Build history of the part. All positions in model axes, mm. Face numbers are marked on the shaded views. A direction names the side the tool comes from. Round coordinates to 2 decimals unless told otherwise and drop trailing zeros. Order: outer loops, then holes, each group sorted by start corner. A loop starts at its lowest first (then second) coordinate and runs counter-clockwise, first axis right, second up. Notation, with made-up numbers: M 55.5,-30 L 100.5,-30 A27 cw 100.5,3 Z; hole C 16.5,-40 d1. An arc over 180 degrees is marked long. One line per item, written item: value. Start each with the question number.
Item 1: Band-saw the part on B-B, the plane x = -107.95. Write the cut outline in (y, z) (3 decimals), then the cut area to 3 significant figures.
Item 2: Two-plate mould, pull along X, no slides. Class the marked faces 6, 7 and 8: +X half, -X half, draft (parallel to the pull), parting line (faces both ways), or undercut.
Item 3: Tool access for the marked faces 1, 2, 3, 4 and 5: list every direction of +Z, -Z, +X, -X, +Y, -Y with a clear straight run to the whole face (end or side of a thin tool).
Item 4: Band-saw the part on D-D, the plane y = 23.5. Write the cut outline in (x, z).
Item 5: Probe L1, parallel to X at y = 203, z = 29; L2, parallel to Y at x = -107.95, z = 28 (3 decimals); L3, parallel to X at y = 208, z = 11. List the from-to ranges inside material, lowest first.
Item 6: Band-saw the part on A-A, the plane y = 203.2. Write the cut outline in (x, z) (3 decimals), then the cut area to 3 significant figures.
Item 7: Pin check, flat tips, straight feed: pin 1 (19 mm diameter, centred on x = 10.5, z = 14.5, fed in from -Y); pin 2 (6 mm diameter, centred on x = -39, z = 7.5, fed in from +Y); pin 3 (1.5 mm diameter, centred on y = 55.5, z = 26.5, fed in from -X). Stop position of each tip, or through.
Item 8: Band-saw the part on C-C, the plane z = 21. Write the cut outline in (x, y) (3 decimals).
```python
from build123d import *

# Parameters (mm, degrees)
F0_W     = 38.1
F0_H     = 38.1
F1_DEPTH = 38.1
F2_R     = 12.7
F4_DEPTH = 38.101


with BuildPart() as f1:
    # F0 (on Top) → F1 (new body)
    with BuildSketch(Plane.XY):
        Polygon((-50.8, 0), (0, 0), (0, 101.6), (0, 139.7), (-50.8, 139.7), (-50.8, 101.6), align=None)
        with Locations((19.05, 120.65)):
            Rectangle(F0_W, F0_H)
        with Locations((-69.85, 120.65)):
            Rectangle(F0_W, F0_H)
        Polygon((38.1, 139.7), (38.1, 101.6), (76.2, 101.6), (76.2, 228.6), (38.1, 228.6), align=None)
        Polygon((-127, 101.6), (-88.9, 101.6), (-88.9, 139.7), (-88.9, 228.6), (-127, 228.6), align=None)
    extrude(amount=F1_DEPTH)

    # F2
    f2_edges = [f1.edges().sort_by_distance(p)[0] for p in [
        (0, 50.8, 38.1),
        (-50.8, 50.8, 38.1),
        (-50.8, 50.8, 0),
        (0, 50.8, 0),
    ]]
    fillet(f2_edges, radius=F2_R)

    # F3 (on face) → F4 (cut, through all)
    with BuildSketch(Plane.XY.offset(38.1)):
        with BuildLine():
            ThreePointArc((-117.475, 203.2), (-107.95, 193.675), (-98.425, 203.2))
            Line((-98.425, 203.2), (-117.475, 203.2))
        make_face()
        with BuildLine():
            Line((66.675, 203.2), (47.625, 203.2))
            ThreePointArc((47.625, 203.2), (57.15, 193.675), (66.675, 203.2))
        make_face()
        with BuildLine():
            ThreePointArc((66.675, 203.2), (57.15, 212.725), (47.625, 203.2))
            Line((47.625, 203.2), (66.675, 203.2))
        make_face()
        with BuildLine():
            Line((-117.475, 203.2), (-98.425, 203.2))
            ThreePointArc((-98.425, 203.2), (-107.95, 212.725), (-117.475, 203.2))
        make_face()
    extrude(amount=-F4_DEPTH, mode=Mode.SUBTRACT)


solid = f1.part
```
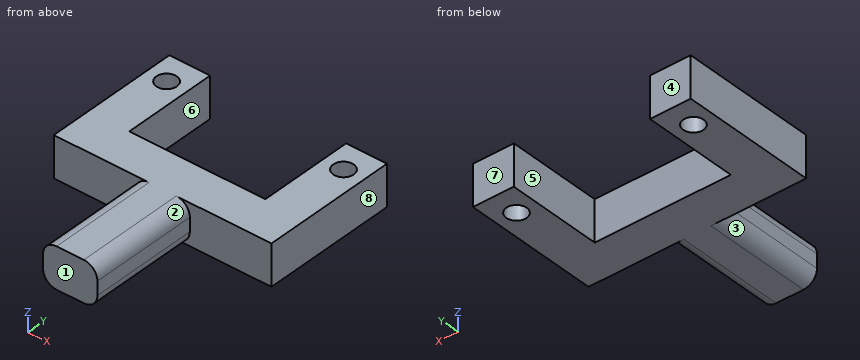
Output:
1. outline: M 101.6,0 L 193.675,0 L 193.675,38.1 L 101.6,38.1 Z; M 212.725,0 L 228.6,0 L 228.6,38.1 L 212.725,38.1 Z
1. area: 4,110 mm²
2. face 6: undercut
2. face 7: draft
2. face 8: +X half
3. face 1: +Z, -Z, +X, -X, -Y
3. face 2: +Z, +X, -Y
3. face 3: -Z, -X, -Y
3. face 4: +Z, -Z, +X, -X, +Y
3. face 5: +Z, -Z, +Y
4. outline: M -50.8,12.7 A12.7 ccw -38.1,0 L -12.7,0 A12.7 ccw 0,12.7 L 0,25.4 A12.7 ccw -12.7,38.1 L -38.1,38.1 A12.7 ccw -50.8,25.4 Z
5. L1: x = -127 to -117.47, -98.43 to -88.9, 38.1 to 47.63, 66.67 to 76.2
5. L2: y = 101.6 to 193.675, 212.725 to 228.6
5. L3: x = -127 to -116.18, -99.72 to -88.9, 38.1 to 48.92, 65.38 to 76.2
6. outline: M -127,0 L -117.475,0 L -117.475,38.1 L -127,38.1 Z; M -98.425,0 L -88.9,0 L -88.9,38.1 L -98.425,38.1 Z; M 38.1,0 L 47.625,0 L 47.625,38.1 L 38.1,38.1 Z; M 66.675,0 L 76.2,0 L 76.2,38.1 L 66.675,38.1 Z
6. area: 1,450 mm²
7. pin 1: stops at y = 101.6
7. pin 2: stops at y = 139.7
7. pin 3: stops at x = -50.8
8. outline: M -127,101.6 L -50.8,101.6 L -50.8,0 L 0,0 L 0,101.6 L 76.2,101.6 L 76.2,228.6 L 38.1,228.6 L 38.1,139.7 L -88.9,139.7 L -88.9,228.6 L -127,228.6 Z; hole C -107.95,203.2 d19.05; hole C 57.15,203.2 d19.05
